Can you work these out from the model? Positions are in its coordinate system, mm. Face numbers are marked on the shaded views. Coordinates: 2 decimals unless noted, no trailing zeros. Order: outer loops, then holes, each group sorted by start corner. A loop starts at its lowest first (then second) coordinate and runs counter-clockwise, first axis right, second up. Notation, with made-up numbers: M 39.5,-19.75 L 97.5,-19.75 A25 cw 97.5,10.25 Z; hole C -32,62 d5. An arc over 180 degrees is marked long. Answer as a JSON object with one key per item and string values.
from build123d import *

# Parameters (mm, degrees)
SKETCH3_W                    = 114
SKETCH3_H                    = 40
BASE_FLANGE1_DEPTH           = 3
EDGE_FLANGE1_STRIP_W         = 13.4732
EDGE_FLANGE1_STRIP_H         = 3
EDGE_FLANGE1_STRIP_CUT_DEPTH = 40
EDGE_FLANGE1_DEPTH           = 40
EDGE_FLANGE2_STRIP_W         = 13.4732
EDGE_FLANGE2_STRIP_H         = 3
EDGE_FLANGE2_STRIP_CUT_DEPTH = 40
EDGE_FLANGE2_DEPTH           = 40
SKETCH11_R                   = 8
SKETCH11_R_2                 = 2
CUT_EXTRUDE1_DEPTH           = 10
CUT_EXTRUDE2_REACH           = 157.592
SKETCH12_R                   = 2


# Sheet-metal steps are written as plain solids
with BuildPart() as part:
    # Sketch3 → Base-Flange1 (new body)
    with BuildSketch(Plane(origin=(0, 0, 0), x_dir=(1, 0, 0), z_dir=(0, 1, 0))):
        Rectangle(SKETCH3_W, SKETCH3_H)
    extrude(amount=-BASE_FLANGE1_DEPTH)

    # Edge-Flange1 strip (across the edge) → Edge-Flange1 strip cut (cut)
    with BuildSketch(Plane(origin=(-57, 0, -20), x_dir=(1, 0, 0), z_dir=(0, 0, 1))):
        with Locations((-6, -1.5)):
            Rectangle(EDGE_FLANGE1_STRIP_W, EDGE_FLANGE1_STRIP_H)
    extrude(amount=EDGE_FLANGE1_STRIP_CUT_DEPTH, mode=Mode.SUBTRACT)

    # Edge-Flange1 section (across the edge) → Edge-Flange1 (add)
    with BuildSketch(Plane(origin=(-57, 0, -20), x_dir=(1, 0, 0), z_dir=(0, 0, 1))):
        with BuildLine():
            Line((-3, 0.7366), (-3, 97))
            Line((-3, 97), (0, 97))
            Line((0, 97), (0, 0.7366))
            ThreePointArc((0, 0.7366), (0.215745145, 0.215745145), (0.7366, 0))
            Line((0.7366, 0), (0.7366, -3))
            ThreePointArc((0.7366, -3), (-1.905575199, -1.905575199), (-3, 0.7366))
        make_face()
    extrude(amount=EDGE_FLANGE1_DEPTH)

    # Edge-Flange2 strip (across the edge) → Edge-Flange2 strip cut (cut)
    with BuildSketch(Plane(origin=(57, 0, 20), x_dir=(-1, 0, 0), z_dir=(0, 0, -1))):
        with Locations((-6, -1.5)):
            Rectangle(EDGE_FLANGE2_STRIP_W, EDGE_FLANGE2_STRIP_H)
    extrude(amount=EDGE_FLANGE2_STRIP_CUT_DEPTH, mode=Mode.SUBTRACT)

    # Edge-Flange2 section (across the edge) → Edge-Flange2 (add)
    with BuildSketch(Plane(origin=(57, 0, 20), x_dir=(-1, 0, 0), z_dir=(0, 0, -1))):
        with BuildLine():
            Line((-3, 0.7366), (-3, 97))
            Line((-3, 97), (0, 97))
            Line((0, 97), (0, 0.7366))
            ThreePointArc((0, 0.7366), (0.215745145, 0.215745145), (0.7366, 0))
            Line((0.7366, 0), (0.7366, -3))
            ThreePointArc((0.7366, -3), (-1.905575199, -1.905575199), (-3, 0.7366))
        make_face()
    extrude(amount=EDGE_FLANGE2_DEPTH)

    # Sketch11 → Cut-Extrude1 (cut)
    with BuildSketch(Plane(origin=(0, -3, 0), x_dir=(-1, 0, 0), z_dir=(0, -1, 0))):
        with Locations(Location((0, 0, 0), (0, 0, 90))):
            Circle(SKETCH11_R)
        with Locations(Location((0, 14, 0), (0, 0, 90))):
            Circle(SKETCH11_R_2)
        with Locations(Location((14, 0, 0), (0, 0, 90))):
            Circle(SKETCH11_R_2)
        with Locations(Location((0, -14, 0), (0, 0, 90))):
            Circle(SKETCH11_R_2)
        with Locations(Location((-14, 0, 0), (0, 0, 90))):
            Circle(SKETCH11_R_2)
    extrude(amount=-CUT_EXTRUDE1_DEPTH, mode=Mode.SUBTRACT)

    # Cut-Extrude2: up to this face of the body (flat: up to its plane)
    cut_extrude2_end = Plane(part.part.faces().sort_by_distance((-60, 48.8683, 0))[0])
    # Sketch12 → Cut-Extrude2 (cut, up to the picked face)
    with BuildSketch(Plane(origin=(60, 0, 0), x_dir=(0, 0, -1), z_dir=(1, 0, 0)), mode=Mode.PRIVATE) as cut_extrude2_sk1:
        with Locations(Location((12.5, 79.674243403, 0), (0, 0, 90))):
            Circle(SKETCH12_R)
    cut_extrude2_tool1 = split(extrude(cut_extrude2_sk1.sketch, amount=-CUT_EXTRUDE2_REACH, mode=Mode.PRIVATE), bisect_by=cut_extrude2_end, keep=Keep.BOTH, mode=Mode.PRIVATE)
    # Sketch12 → Cut-Extrude2 (cut, up to the picked face)
    with BuildSketch(Plane(origin=(60, 0, 0), x_dir=(0, 0, -1), z_dir=(1, 0, 0)), mode=Mode.PRIVATE) as cut_extrude2_sk2:
        with Locations(Location((12.5, 90.674243403, 0), (0, 0, 90))):
            Circle(SKETCH12_R)
    cut_extrude2_tool2 = split(extrude(cut_extrude2_sk2.sketch, amount=-CUT_EXTRUDE2_REACH, mode=Mode.PRIVATE), bisect_by=cut_extrude2_end, keep=Keep.BOTH, mode=Mode.PRIVATE)
    # Sketch12 → Cut-Extrude2 (cut, up to the picked face)
    with BuildSketch(Plane(origin=(60, 0, 0), x_dir=(0, 0, -1), z_dir=(1, 0, 0)), mode=Mode.PRIVATE) as cut_extrude2_sk3:
        with Locations(Location((-12.5, 79.674243403, 0), (0, 0, 90))):
            Circle(SKETCH12_R)
    cut_extrude2_tool3 = split(extrude(cut_extrude2_sk3.sketch, amount=-CUT_EXTRUDE2_REACH, mode=Mode.PRIVATE), bisect_by=cut_extrude2_end, keep=Keep.BOTH, mode=Mode.PRIVATE)
    # Sketch12 → Cut-Extrude2 (cut, up to the picked face)
    with BuildSketch(Plane(origin=(60, 0, 0), x_dir=(0, 0, -1), z_dir=(1, 0, 0)), mode=Mode.PRIVATE) as cut_extrude2_sk4:
        with Locations(Location((-12.5, 90.674243403, 0), (0, 0, 90))):
            Circle(SKETCH12_R)
    cut_extrude2_tool4 = split(extrude(cut_extrude2_sk4.sketch, amount=-CUT_EXTRUDE2_REACH, mode=Mode.PRIVATE), bisect_by=cut_extrude2_end, keep=Keep.BOTH, mode=Mode.PRIVATE)
    add(cut_extrude2_tool1.solids().sort_by(Axis((60, 79.674243, -12.5), (-1, 0, 0)))[0], mode=Mode.SUBTRACT)
    add(cut_extrude2_tool2.solids().sort_by(Axis((60, 90.674243, -12.5), (-1, 0, 0)))[0], mode=Mode.SUBTRACT)
    add(cut_extrude2_tool3.solids().sort_by(Axis((60, 79.674243, 12.5), (-1, 0, 0)))[0], mode=Mode.SUBTRACT)
    add(cut_extrude2_tool4.solids().sort_by(Axis((60, 90.674243, 12.5), (-1, 0, 0)))[0], mode=Mode.SUBTRACT)


solid = part.part
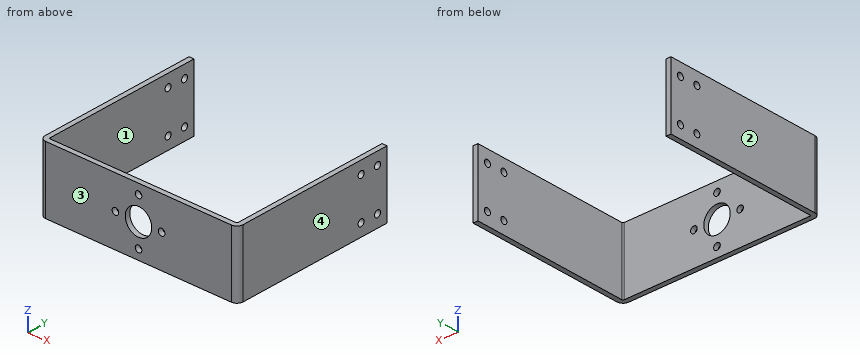
Item 1: I want a section at A-A, the plane z = 0. Write out the boundary of the cut face in (x, y).
Answers follow:
{"outline": "M -60,0.74 A3.74 ccw -56.26,-3 L -16,-3 L -16,0 L -56.26,0 A0.74 cw -57,0.74 L -57,97 L -60,97 Z; M -12,-3 L -8,-3 L -8,0 L -12,0 Z; M 8,-3 L 12,-3 L 12,0 L 8,0 Z; M 16,-3 L 56.26,-3 A3.74 ccw 60,0.74 L 60,97 L 57,97 L 57,0.74 A0.74 cw 56.26,0 L 16,0 Z"}
Item 2: I want a section at B-B, the plane y = 53. Write out the boundary of the cut face in (x, z), plus the area to 3 significant figures.
Answers follow:
{"outline": "M -60,-20 L -57,-20 L -57,20 L -60,20 Z; M 57,-20 L 60,-20 L 60,20 L 57,20 Z", "area": "240 mm^2"}
Item 3: I want a section at C-C, the plane x = 14. Write out the boundary of the cut face in (y, z).
Answers follow:
{"outline": "M -3,-20 L 0,-20 L 0,-2 L -3,-2 Z; M -3,2 L 0,2 L 0,20 L -3,20 Z"}
Item 4: Please list where these lines run through material, in increasing order: line 1 (X direction, y = 69, z = 7); line 2 (Y direction, x = 58, z = 12); line 3 (X direction, y = -1.75, z = 0).
Answers follow:
{"line 1": "x = -60 to -57, 57 to 60", "line 2": "y = -2.57 to 77.74, 81.61 to 88.74, 92.61 to 97", "line 3": "x = -59.05 to -16, -12 to -8, 8 to 12, 16 to 59.05"}
Item 5: I want a section at D-D, the plane x = 35. Write out the boundary of the cut face in (y, z).
Answers follow:
{"outline": "M -3,-20 L 0,-20 L 0,20 L -3,20 Z"}
Item 6: If we mould it in two halves opening along X, with no side actions, what happens to the marked faces 1, 2, 3 and 4? For each: pulls with the +X half, pulls with the -X half, needs draft (parallel to the pull), parting line crosses it, or undercut.
Answers follow:
{"face 1": "undercut", "face 2": "pulls with the -X half", "face 3": "needs draft", "face 4": "pulls with the +X half"}
Item 7: I'm going to push flat-ended pins straight in: pin 1 (6.5 mm diameter, centred on y = 79.67, z = 12.5, fed in from -X); pin 2 (12 mm diameter, centred on x = 2, z = -2, fed in from +Y). Where does each tip first touch, or does it pass through?
Answers follow:
{"pin 1": "stops at x = -60", "pin 2": "stops at y = 0"}
